Part model, mm, in its own coordinate system. A direction names the side the tool comes from. Give positions to 0.01 mm unless a question says otherwise; leave off trailing zeros. Order: outer loops, then holes, each group sorted by start corner. A loop starts at its lowest first (then second) coordinate and runs counter-clockwise, first axis right, second up. Notation, with made-up numbers: (70, -2.5) -> (102, -2.5) arc R7 ccw to (102, 1.5) -> close; hole circle Ø4 at (-4, 27.25). An arc over 180 degrees is marked (long way). Write item = value, one per line. Start each with the question number.
(1) Saw through at B-B, the plane x = 0. List the corners of the cut face in (y, z).
(2) Flat gauge pins, fed straight in: pin 1 (0.5 mm diameter, centred on x = 11.5, y = 1, fed in from -Z) (3 decimals); pin 2 (0.8 mm diameter, centred on y = 1, z = 16.5, fed in from +X); pin 3 (0.5 mm diameter, centred on x = -12, y = 1, fed in from +Z) (3 decimals). Where does each tip first touch, or does it go through?
(3) Which spindle directions (+Z, -Z, +X, -X, +Y, -Y) get a long thin tool onto all of the face, cutting with end or side? Do faces 4 (the flat face through (11.112, 1, -17)), 5 (the flat face through (-12, 1, -9.525)), 6 (the flat face through (12, 1, 9.525)), 7 (the flat face through (-12, 1, 9.525)). Say none if no direction does.
(4) Saw through at C-C, the plane x = 7. List the corners of the cut face in (y, z).
(5) Probe line 1 along Z through (x, y) = (11.75, 0.45) (3 decimals); line 2 along X through (y, z) = (1.25, -12.5); line 3 along Z through (x, y) = (-8.25, 0.55). List the from-to ranges inside material, lowest first. Write a range as from..to.
(6) Two-plate mould, pull along X, no slides. Class faces 1 (the cylindrical face through (-0.24, 0.78, 7.94)), 2 (the flat face through (12.7, 1, 0)), 3 (the flat face through (0, 1.588, -8)): pulls with the +X half, pulls with the -X half, needs draft (parallel to the pull), parting line crosses it, or undercut.
from build123d import *

# Parameters (mm, degrees)
SKETCH1_W           = 1.5875
SKETCH1_H           = 19.05
BOSS_EXTRUDE1_DEPTH = 1.5875


with BuildPart() as part:
    # Sketch1 → Boss-Extrude1 (new body)
    with BuildSketch(Plane(origin=(0, 0, 0), x_dir=(1, 0, 0), z_dir=(0, 1, 0))):
        with BuildLine():
            Line((11.1125, 9.525), (11.1125, 25.4))
            Line((11.1125, 25.4), (-11.1125, 25.4))
            Line((-11.1125, 25.4), (-11.1125, 9.525))
            Line((-11.1125, 9.525), (-11.1125, -9.525))
            Line((-11.1125, -9.525), (-11.1125, -19.05))
            ThreePointArc((-11.1125, -19.05), (0, -7.9375), (11.1125, -19.05))
            Line((11.1125, -19.05), (11.1125, -9.525))
            Line((11.1125, -9.525), (11.1125, 9.525))
        make_face()
        with Locations((11.90625, 0)):
            Rectangle(SKETCH1_W, SKETCH1_H)
        with Locations((-11.90625, 0)):
            Rectangle(SKETCH1_W, SKETCH1_H)
    extrude(amount=BOSS_EXTRUDE1_DEPTH)


solid = part.part
Results list:
q1.outline = (0, -25.4) -> (1.59, -25.4) -> (1.59, 7.94) -> (0, 7.94) -> close
q2.pin_1 = -9.525
q2.pin_2 = 11.11
q2.pin_3 = 9.525
q3.face_4 = -Z, +X, +Y, -Y
q3.face_5 = -Z, -X, +Y, -Y
q3.face_6 = +Z, +X, +Y, -Y
q3.face_7 = +Z, -X, +Y, -Y
q4.outline = (0, -25.4) -> (1.59, -25.4) -> (1.59, 10.42) -> (0, 10.42) -> close
q5.line_1 = -9.525..9.525
q5.line_2 = -11.11..11.11
q5.line_3 = -25.4..11.61
q6.face_1 = undercut
q6.face_2 = pulls with the +X half
q6.face_3 = needs draft
